Design review of the part built by this model. Coordinates are the model's own, in mm. Round coordinates to 2 decimals unless told otherwise and drop trailing zeros. Loops run counter-clockwise (first coordinate to the right, second up) from the corner with the lowest first, then second, coordinate; pieces in that order, holes last. Notation, with made-up numbers: (43, 55) - (69, 55) arc R26 cw to (69, 80) - close; hole circle Ø3 at (-39, 30.5). An arc over 180 degrees is marked (long way). Answer as CSV lines item,"result". Start each with the question number.
(1) Consider section C-C (z = -34). Give the boundary of the cut face in (x, y).
(2) Consider section A-A (z = -20). Give the boundary of the cut face in (x, y), and give its area (3 significant figures).
(3) For P1, Ø2.5, axis at x = 14.8, z = -6, coming from the +Y side, flat-tipped, find the tip position at first contact; note if it passes through.
(4) Consider section B-B (x = -24.69). Give the boundary of the cut face in (y, z), and give its area (3 significant figures).
(5) Consider section D-D (y = -0.5). Count the separate pieces of the cut face and the enclosed holes in it, and give its area (3 significant figures).
(6) Mouldability with a two-part tool opening along Z and no side actions: class faces 1 (the flat face through (-24.945, -0.74, -5.583)), 2 (the flat face through (-24.63, -0.74, -34.57)), 3 (the cylindrical face through (13.8, -0.7, -5.7)) as released by +Z, released by -Z, zero draft, split by the parting line, or undercut.
(7) Wall thickness on L1, parallel to X at y = -1.25, z = -33.5; L2, parallel to Z at x = 14, y = -1.3; L3, parallel to X at y = -0.3, z = -22: over which ranges is each line inside the solid? List them lowest first.
Autodesk Inventor part; units mm, degrees
ref_plane "YZ Plane" through (0, 0, 0) normal (1, 0, 0) x (0, 1, 0)
ref_plane "XZ Plane" through (0, 0, 0) normal (0, 1, 0) x (-1, 0, 0)
ref_plane "XY Plane" through (0, 0, 0) normal (0, 0, 1) x (1, 0, 0)
sketch "Sketch1" plane through (0, 0, 0) normal (0, 1, 0) x (-1, 0, 0)
  line L0 (-0.4496, -40) -> (-0.4496, 0)
  line L1 (-27.6589, 0) -> (-27.6589, -40)
  circle A0 centre (-5.3993, -34) radius 1.05
  circle A1 centre (-14.8043, -34) radius 1.05
  circle A2 centre (-24.2093, -34) radius 1.05
  circle A3 centre (-24.2093, -6) radius 1.05
  circle A4 centre (-14.8043, -6) radius 1.05
  circle A5 centre (-5.3993, -6) radius 1.05
  circle A6 centre (-59.7986, -20) radius 2.55
  circle A7 centre (31.69, -20) radius 2.6
  circle A8 centre (24.69, -20) radius 1.05
  circle A9 centre (31.69, -13) radius 1.05
  circle A10 centre (31.69, -27) radius 1.05
  circle A11 centre (38.69, -20) radius 1.05
  line L2 (36.0744, -11.0124) -> (13.5, 0)
  line L3 (-41.6086, 0) -> (-64.183, -11.0124)
  line L4 (13.5, -40) -> (36.0744, -28.9876)
  line L5 (-64.183, -28.9876) -> (-41.6086, -40)
  arc A12 (36.0744, -28.9876) -> (36.0744, -11.0124) centre (31.69, -20) ccw
  arc A13 (-64.183, -11.0124) -> (-64.183, -28.9876) centre (-59.7986, -20) ccw
  line L6 (-41.6086, 0) -> (13.5, 0)
  line L7 (13.5, -40) -> (-41.6086, -40)
  line L8 (-28.1086, -40) -> (-28.1086, 0)
  line L9 (-27.2093, 0) -> (-27.2093, -40)
  line L10 (-0.8993, -40) -> (-0.8993, 0)
  line L11 (0, 0) -> (0, -40)
extrude "Extrusion1" add sketch "Sketch1" against normal blind 1.5
properties part number "CAM_axis_6_supplement_frame"
Determined:
1,outline,"(-25.8, -1.5) - (4.35, -1.5) - (4.35, 0) - (-25.8, 0) - close; (6.45, -1.5) - (13.75, -1.5) - (13.75, 0) - (6.45, 0) - close; (15.85, -1.5) - (23.16, -1.5) - (23.16, 0) - (15.85, 0) - close; (25.26, -1.5) - (53.91, -1.5) - (53.91, 0) - (25.26, 0) - close"
2,outline,"(-41.69, -1.5) - (-39.74, -1.5) - (-39.74, 0) - (-41.69, 0) - close; (-37.64, -1.5) - (-34.29, -1.5) - (-34.29, 0) - (-37.64, 0) - close; (-29.09, -1.5) - (-25.74, -1.5) - (-25.74, 0) - (-29.09, 0) - close; (-23.64, -1.5) - (57.25, -1.5) - (57.25, 0) - (-23.64, 0) - close; (62.35, -1.5) - (69.8, -1.5) - (69.8, 0) - (62.35, 0) - close"
2,area,"145 mm^2"
3,P1,"stops at y = 0"
4,outline,"(-1.5, -34.54) - (0, -34.54) - (0, -21.05) - (-1.5, -21.05) - close; (-1.5, -18.95) - (0, -18.95) - (0, -5.46) - (-1.5, -5.46) - close"
4,area,"40.5 mm^2"
5,separate pieces,"1"
5,enclosed holes,"12"
5,area,"3,580 mm^2"
6,face 1,"released by +Z"
6,face 2,"released by -Z"
6,face 3,"undercut"
7,L1,"x = -26.82 to 4.48, 6.32 to 13.88, 15.73 to 23.29, 25.13 to 54.93"
7,L2,"z = -40 to -34.67, -33.33 to -6.67, -5.33 to 0"
7,L3,"x = -41.49 to -33.35, -30.03 to 58.22, 61.38 to 69.6"
